```python
from build123d import *

# Parameters (mm, degrees)
SKETCH2_W           = 140
SKETCH2_H           = 100
BOSS_EXTRUDE1_DEPTH = 10
SKETCH3_R           = 3.5
BOSS_EXTRUDE2_DEPTH = 30
FILLET1_R           = 8
SKETCH4_W           = 5
SKETCH4_H           = 41.8
CUT_EXTRUDE1_DEPTH  = 30


with BuildPart() as part:
    # Sketch2 → Boss-Extrude1 (new body)
    with BuildSketch(Plane(origin=(0, 0, 0), x_dir=(0, 0, -1), z_dir=(1, 0, 0))):
        Rectangle(SKETCH2_W, SKETCH2_H)
    extrude(amount=BOSS_EXTRUDE1_DEPTH)

    # Sketch3 → Boss-Extrude2 (add)
    with BuildSketch(Plane.ZY):
        with Locations(Location((-65, 31.6267322, 0), (0, 0, 180))):
            Circle(SKETCH3_R)
        with Locations(Location((-65, -8.3732678, 0), (0, 0, 180))):
            Circle(SKETCH3_R)
        with Locations(Location((65, 31.6267322, 0), (0, 0, 180))):
            Circle(SKETCH3_R)
        with Locations(Location((65, -8.3732678, 0), (0, 0, 180))):
            Circle(SKETCH3_R)
    extrude(amount=BOSS_EXTRUDE2_DEPTH)

    # Fillet1
    fillet1_edges = [part.edges().sort_by_distance(p)[0] for p in [
        (10, 0, -70),
        (10, 0, 70),
    ]]
    fillet(fillet1_edges, radius=FILLET1_R)

    # Sketch4 → Cut-Extrude1 (cut)
    with BuildSketch(Plane(origin=(10, 0, 0), x_dir=(0, 0, -1), z_dir=(1, 0, 0))):
        with Locations((18.5, 1.2)):
            Rectangle(SKETCH4_W, SKETCH4_H)
        with Locations((28.5, 1.2)):
            Rectangle(SKETCH4_W, SKETCH4_H)
        with Locations((-1.5, 1.2)):
            Rectangle(SKETCH4_W, SKETCH4_H)
        with Locations((8.5, 1.2)):
            Rectangle(SKETCH4_W, SKETCH4_H)
        with Locations((-21.5, 1.2)):
            Rectangle(SKETCH4_W, SKETCH4_H)
        with Locations((-11.5, 1.2)):
            Rectangle(SKETCH4_W, SKETCH4_H)
    extrude(amount=-CUT_EXTRUDE1_DEPTH, mode=Mode.SUBTRACT)


solid = part.part
```
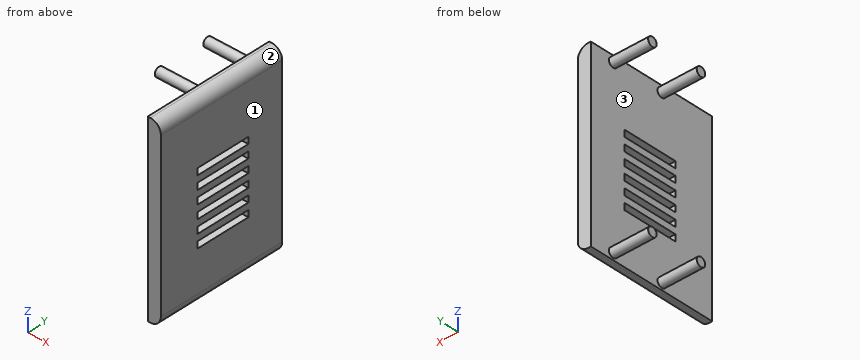
The model under review builds one solid part; all positions refer to its coordinate system, in mm. Face numbers are marked on the shaded views. Round coordinates to 2 decimals unless told otherwise and drop trailing zeros. Order: outer loops, then holes, each group sorted by start corner. A loop starts at its lowest first (then second) coordinate and runs counter-clockwise, first axis right, second up. Notation, with made-up numbers: (-14.75, 42) -> (21.25, 42) arc R31 ccw to (21.25, 69) -> close; hole circle Ø2 at (-26, 26.5). An arc over 180 degrees is marked (long way). Use a Markdown table: item, result.
Q1. We need section C-C on z = 65. Write out the cut boundary in (x, y), then the cut area to 3 significant figures.
Values:
| item | result |
|---|---|
| outline | (-30, -11.87) -> (0, -11.87) -> (0, -50) -> (9.42, -50) -> (9.42, 50) -> (0, 50) -> (0, 35.13) -> (-30, 35.13) -> (-30, 28.13) -> (0, 28.13) -> (0, -4.87) -> (-30, -4.87) -> close |
| area | 1,360 mm^2 |
Q2. We need section D-D on y = 44. Write out the cut boundary in (x, z), then the cut area to 3 significant figures.
Values:
| item | result |
|---|---|
| outline | (0, -70) -> (2, -70) arc R8 ccw to (10, -62) -> (10, 62) arc R8 ccw to (2, 70) -> (0, 70) -> close |
| area | 1,370 mm^2 |
Q3. We need section B-B on x = -24. Write out the cut boundary in (y, z).
Values:
| item | result |
|---|---|
| outline | circle Ø7 at (-8.37, -65); circle Ø7 at (-8.37, 65); circle Ø7 at (31.63, -65); circle Ø7 at (31.63, 65) |
Q4. We need section A-A on y = 12.5. State how many separate pieces and enclosed holes the cut face has, then the cut area to 3 significant figures.
Values:
| item | result |
|---|---|
| separate pieces | 7 |
| enclosed holes | 0 |
| area | 1,070 mm^2 |
Q5. Mouldability with a two-part tool opening along Z and no side actions: class the marked faces 1, 2 and 3 as +Z half, -Z half, draft (parallel to the pull), parting line (faces both ways), or undercut.
Values:
| item | result |
|---|---|
| face 1 | draft |
| face 2 | +Z half |
| face 3 | undercut |
Q6. For line 1 (X direction, y = 35.5, z = -62); line 2 (Z direction, x = -21, y = 34.5); line 3 (Y direction, x = -25, z = -63.5), list the stretches that pass through material, from the lowest coordinate up.
Values:
| item | result |
|---|---|
| line 1 | x = 0 to 10 |
| line 2 | z = -67 to -63, 63 to 67 |
| line 3 | y = -11.54 to -5.21, 28.46 to 34.79 |
Q7. Clearance check with flat-ended pins moving along their axes: P1, Ø10, axis at y = -3.5, z = -31, coming from the -X side; P2, Ø3, axis at x = 7, y = -9, coming from the +Z side; P3, Ø3, axis at x = 6, y = 2.5, coming from the -Z side. State where each tip first meets the part, or that it passes through.
Values:
| item | result |
|---|---|
| P1 | stops at x = 0 |
| P2 | stops at z = 69.19 |
| P3 | stops at z = -69.6 |
